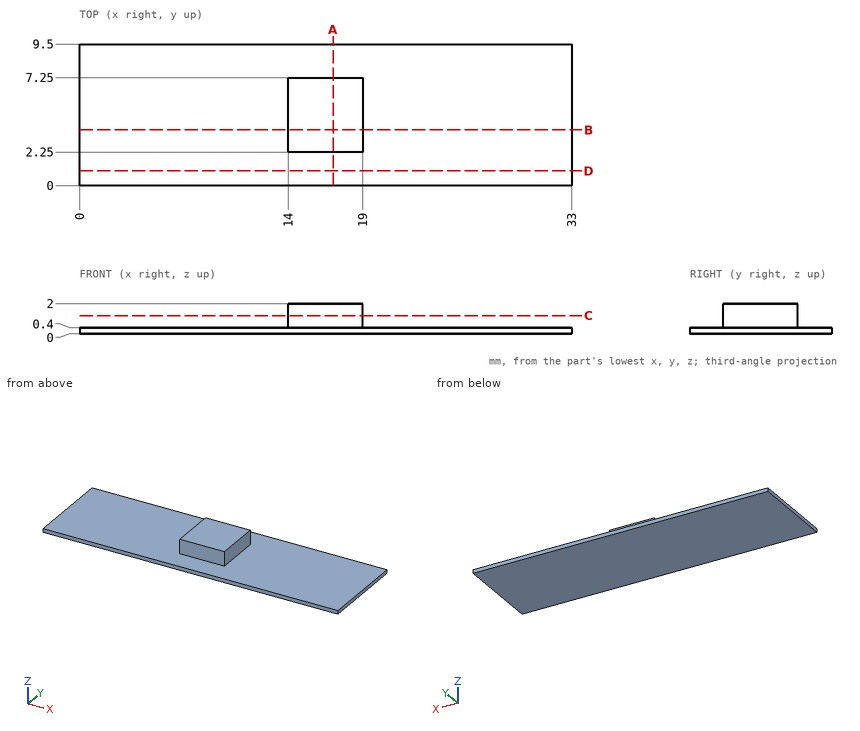
The figure shows three views and two pictorial views of one solid part (mm, origin at its lowest corner). Answer the questions. Round coordinates to 2 decimals unless told otherwise and drop trailing zeros. Order: outer loops, then holes, each group sorted by start corner. A loop starts at its lowest first (then second) coordinate and runs counter-clockwise, first axis right, second up. Notation, with made-up numbers: (-13, 39.25) -> (4, 39.25) arc R24 ccw to (4, 50.25) -> close; hole circle Ø6 at (61, 12.25). An arc over 180 degrees is marked (long way). Put each result on its own line as item: value.
Q1. Consider line 1 along Z through (x, y) = (6, 8); line 2 along X through (y, z) = (6, 1.6); line 3 along Y through (x, z) = (18.5, 1.95). Determine where each line is inside the solid, lowest interval first.
Results list:
line 1: 0 to 0.4
line 2: 14 to 19
line 3: 2.25 to 7.25
Q2. Section D-D, the plane y = 1 is taken. Write down the section's boundary in (x, z).
Results list:
outline: (0, 0) -> (33, 0) -> (33, 0.4) -> (0, 0.4) -> close
Q3. Section B-B, the plane y = 3.75 is taken. Write down the section's boundary in (x, z).
Results list:
outline: (0, 0) -> (33, 0) -> (33, 0.4) -> (19, 0.4) -> (19, 2) -> (14, 2) -> (14, 0.4) -> (0, 0.4) -> close
Q4. Section C-C, the plane z = 1.2 is taken. Write down the section's boundary in (x, y), and give its area (3 significant figures).
Results list:
outline: (14, 2.25) -> (19, 2.25) -> (19, 7.25) -> (14, 7.25) -> close
area: 25.0 mm^2
Q5. Section A-A, the plane x = 17 is taken. Write down the section's boundary in (y, z).
Results list:
outline: (0, 0) -> (9.5, 0) -> (9.5, 0.4) -> (7.25, 0.4) -> (7.25, 2) -> (2.25, 2) -> (2.25, 0.4) -> (0, 0.4) -> close
Q6. Each of these flat-tipped pins is pushed along its axis until it touches: P1, Ø1, axis at x = 19.5, y = 2, coming from the +Z side; P2, Ø0.5, axis at y = 5.5, z = 1.5, coming from the +X side; P3, Ø1, axis at y = 3, z = 1.5, coming from the -X side. Where does it stop, or does it pass through?
Results list:
P1: z = 0.4
P2: x = 19
P3: x = 14
